from build123d import *

# Parameters (mm, degrees)
SKETCH1_W            = 60
SKETCH1_H            = 20
BOSS_EXTRUDE1_DEPTH  = 2.54
SKETCH2_R            = 3.85
EYESHAFT_HOLES_DEPTH = 10
SKETCH5_W            = 4.8
SKETCH5_H            = 2
FRONT_LEGS_DEPTH     = 20
SKETCH7_W            = 10
SKETCH7_H            = 3.2
BACK_LEGS_DEPTH      = 20
FILLET2_R            = 5


with BuildPart() as part:
    # Sketch1 → Boss-Extrude1 (new body)
    with BuildSketch(Plane(origin=(0, 0, 0), x_dir=(1, 0, 0), z_dir=(0, 1, 0))):
        Rectangle(SKETCH1_W, SKETCH1_H)
    extrude(amount=BOSS_EXTRUDE1_DEPTH)

    # Sketch2 → Eyeshaft holes (cut)
    with BuildSketch(Plane(origin=(0, 2.54, 0), x_dir=(1, 0, 0), z_dir=(0, 1, 0))):
        with Locations(Location((-22, -4, 0), (0, 0, 270))):
            Circle(SKETCH2_R)
        with Locations(Location((22, -4, 0), (0, 0, 270))):
            Circle(SKETCH2_R)
    extrude(amount=-EYESHAFT_HOLES_DEPTH, mode=Mode.SUBTRACT)

    # Sketch5 → Front Legs (add)
    with BuildSketch(Plane.XZ):
        with Locations((-12, 4)):
            Rectangle(SKETCH5_W, SKETCH5_H)
        with Locations((12, 4)):
            Rectangle(SKETCH5_W, SKETCH5_H)
    extrude(amount=FRONT_LEGS_DEPTH)

    # Sketch7 → Back legs (add)
    with BuildSketch(Plane.XZ):
        with Locations((-14, -4.45)):
            Rectangle(SKETCH7_W, SKETCH7_H)
        with Locations((14, -4.45)):
            Rectangle(SKETCH7_W, SKETCH7_H)
    extrude(amount=BACK_LEGS_DEPTH)

    # Fillet2
    fillet2_edges = [part.edges().sort_by_distance(p)[0] for p in [
        (30, 1.27, 10),
        (-30, 1.27, 10),
        (-30, 1.27, -10),
        (30, 1.27, -10),
    ]]
    fillet(fillet2_edges, radius=FILLET2_R)


solid = part.part
Geometry: final body of the model. Coordinates: model frame, mm. A direction names the side the tool comes from. Coordinates: 2 decimals unless noted, no trailing zeros. Write each loop counter-clockwise with the first axis right and the second up, starting at its lowest first coordinate (ties: lowest second). Pieces come first, ordered by that corner, then holes. Notation, with made-up numbers: (-4.5, 52.5) - (30.5, 52.5) arc R19 ccw to (30.5, 70.5) - close; hole circle Ø10 at (18.25, 73). An arc over 180 degrees is marked (long way). Return JSON: item names as keys, results as strings.
Item 1: Line query: L1, parallel to X at y = 1.95, z = 4; L2, parallel to Z at x = 13, y = -15; L3, parallel to Y at x = -26.5, z = 7.25. Output: solid intervals per line, ascending.
Completed:
{"L1": "x = -30 to -25.85, -18.15 to 18.15, 25.85 to 30", "L2": "z = -6.05 to -2.85, 3 to 5", "L3": "y = 0 to 2.54"}
Item 2: Pull-direction query (X, two-part tool) for faces 1 (the face through (-30, 1, 0)), 2 (the face through (12, -10, 3)), 3 (the face through (9.6, -10, 4)), 4 (the face through (-9.6, -10, 4)); classes: +X half, -X half, draft (parallel to the pull), parting line (faces both ways), or undercut.
Completed:
{"face 1": "-X half", "face 2": "draft", "face 3": "undercut", "face 4": "undercut"}
Item 3: Section query D-D (z = -4). Output: boundary loops of the cut face in (x, y), and give its area (3 significant figures).
Completed:
{"outline": "(-30, 0) - (-19, 0) - (-19, -20) - (-9, -20) - (-9, 0) - (9, 0) - (9, -20) - (19, -20) - (19, 0) - (30, 0) - (30, 2.54) - (-30, 2.54) - close", "area": "552 mm2"}
Item 4: Section query A-A (x = -22). Output: boundary loops of the cut face in (y, z), and give its area (3 significant figures).
Completed:
{"outline": "(0, -10) - (2.54, -10) - (2.54, 0.15) - (0, 0.15) - close; (0, 7.85) - (2.54, 7.85) - (2.54, 10) - (0, 10) - close", "area": "31.2 mm2"}
Item 5: Reachability of faces 5 (the face through (14, -10, -6.05)), 6 (the face through (19, -10, -4)), 7 (the face through (-14, -10, -2.85)) from +Z, -Z, +X, -X, +Y, -Y: full face, straight path, thin tool, end or side. Return the list, or none.
Completed:
{"face 5": "-Z, +X, -X, -Y", "face 6": "+Z, -Z, +X, -Y", "face 7": "+X, -X, -Y"}
Item 6: Pin query (flat end, axial travel): pin 1 Ø1.6 at (y, z) = (-14, -4.5) entering from +X; pin 2 Ø0.6 at (y, z) = (-13.5, 3.5) entering from +X; pin 3 Ø4 at (x, y) = (-8.5, -9.5) entering from -Z; pin 4 Ø4 at (x, y) = (-3.5, -0.5) entering from +Z. Return the tip coordinate at first contact, or that it passes through.
Completed:
{"pin 1": "stops at x = 19", "pin 2": "stops at x = 14.4", "pin 3": "stops at z = -6.05", "pin 4": "stops at z = 10"}
Item 7: Section query C-C (z = 4). Output: boundary loops of the cut face in (x, y), and give its area (3 significant figures).
Completed:
{"outline": "(-30, 0) - (-25.85, 0) - (-25.85, 2.54) - (-30, 2.54) - close; (-18.15, 0) - (-14.4, 0) - (-14.4, -20) - (-9.6, -20) - (-9.6, 0) - (9.6, 0) - (9.6, -20) - (14.4, -20) - (14.4, 0) - (18.15, 0) - (18.15, 2.54) - (-18.15, 2.54) - close; (25.85, 0) - (30, 0) - (30, 2.54) - (25.85, 2.54) - close", "area": "305 mm2"}
Item 8: Section query B-B (y = -3.5). Output: boundary loops of the cut face in (x, z).
Completed:
{"outline": "(-19, -6.05) - (-9, -6.05) - (-9, -2.85) - (-19, -2.85) - close; (-14.4, 3) - (-9.6, 3) - (-9.6, 5) - (-14.4, 5) - close; (9, -6.05) - (19, -6.05) - (19, -2.85) - (9, -2.85) - close; (9.6, 3) - (14.4, 3) - (14.4, 5) - (9.6, 5) - close"}
